The listing builds one solid part. Answer for the finished solid, in the listing's coordinates (mm). Round coordinates to 2 decimals unless told otherwise and drop trailing zeros. Order: outer loops, then holes, each group sorted by start corner. A loop starts at its lowest first (then second) coordinate and runs counter-clockwise, first axis right, second up. Notation, with made-up numbers: (71.5, 64.5) - (86.5, 64.5) arc R22 ccw to (86.5, 103.5) - close; hole circle Ø1 at (34, 25.25). An arc over 180 degrees is marked (long way). One line per item, written item: value. Start each with the question number.
1. Section C-C, the plane z = 0.9 is taken. Give the vertices of the cut face in (x, y).
2. Straight lines are drawn through the part: line 1 (X direction, y = 29, z = 0.9); line 2 (Y direction, x = 39.5, z = 0.95); line 3 (Y direction, x = 73.5, z = 0.2). For each, find the intervals that lie inside material, in ascending order.
3. Section D-D, the plane y = 59 is taken. Give the vertices of the cut face in (x, z), then the cut area to 3 significant figures.
4. Section B-B, the plane y = 36 is taken. Give the vertices of the cut face in (x, z), then the cut area to 3 significant figures.
5. Section A-A, the plane x = 40 is taken. Give the vertices of the cut face in (y, z).
6. Flat-ended cylindrical pins translate along their axes: P1, Ø0.8, axis at y = 61, z = 0.5, coming from the +X side; P2, Ø1.5, axis at x = 45.5, y = 37.5, coming from the -Z side; P3, Ø0.5, axis at y = 67, z = 0.5, coming from the -X side. Find the tip coordinate at first contact, or state that the pin passes through.
from build123d import *

# Parameters (mm, degrees)
BOARD_W             = 22.5
BOARD_H             = 26.72
BOSS_EXTRUDE2_DEPTH = 1.6


with BuildPart() as part:
    # BOARD → Boss-Extrude2 (new body)
    with BuildSketch(Plane.XY):
        with BuildLine():
            Line((78.158087673, 14.315192257), (83.26046847, 8.69))
            Line((83.26046847, 8.69), (83.26046847, 0.03))
            Line((83.26046847, 0.03), (0.28, 0.03))
            Line((0.28, 0.03), (0.28, 8.69))
            Line((0.28, 8.69), (5.37370372, 14.323050696))
            ThreePointArc((5.37370372, 14.323050696), (8.254635545, 18.990143234), (9.27, 24.38))
            Line((9.27, 24.38), (9.27, 91.540000744))
            ThreePointArc((9.27, 91.540000744), (9.567594313, 92.239511842), (10.270147398, 92.529851835))
            Line((10.270147398, 92.529851835), (73.290147398, 92.529851835))
            ThreePointArc((73.290147398, 92.529851835), (73.989702799, 92.232361682), (74.280147398, 91.529851835))
            Line((74.280147398, 91.529851835), (74.280147398, 24.369851835))
            ThreePointArc((74.280147398, 24.369851835), (75.287357034, 18.983155173), (78.158087673, 14.315192257))
        make_face()
        with Locations((36.93, 39.42)):
            Rectangle(BOARD_W, BOARD_H, mode=Mode.SUBTRACT)
    extrude(amount=BOSS_EXTRUDE2_DEPTH)


solid = part.part
Answer list:
1. outline: (0.28, 0.03) - (83.26, 0.03) - (83.26, 8.69) - (78.16, 14.32) arc R15.04 cw to (74.28, 24.37) - (74.28, 91.53) arc R1 ccw to (73.29, 92.53) - (10.27, 92.53) arc R1 ccw to (9.27, 91.54) - (9.27, 24.38) arc R15.04 cw to (5.37, 14.32) - (0.28, 8.69) - close; hole (25.68, 26.06) - (48.18, 26.06) - (48.18, 52.78) - (25.68, 52.78) - close
2. line 1: x = 9.27 to 25.68, 48.18 to 74.28
2. line 2: y = 0.03 to 26.06, 52.78 to 92.53
2. line 3: y = 0.03 to 92.5
3. outline: (9.27, 0) - (74.28, 0) - (74.28, 1.6) - (9.27, 1.6) - close
3. area: 104 mm²
4. outline: (9.27, 0) - (25.68, 0) - (25.68, 1.6) - (9.27, 1.6) - close; (48.18, 0) - (74.28, 0) - (74.28, 1.6) - (48.18, 1.6) - close
4. area: 68.0 mm²
5. outline: (0.03, 0) - (26.06, 0) - (26.06, 1.6) - (0.03, 1.6) - close; (52.78, 0) - (92.53, 0) - (92.53, 1.6) - (52.78, 1.6) - close
6. P1: stops at x = 74.28
6. P2: passes through
6. P3: stops at x = 9.27
